```python
from build123d import *

# Parameters (mm, degrees)
SKETCH1_W           = 105
SKETCH1_H           = 530
BOSS_EXTRUDE1_DEPTH = 7.5
LPATTERN1_COUNT     = 4
LPATTERN1_PITCH     = 25


# Read off the part's stored shape, not the designer's step: Mirror1
with BuildPart() as part:
    # Sketch1 → Boss-Extrude1 (new, symmetric)
    with BuildSketch(Plane(origin=(0, 0, 0), x_dir=(0, -1, 0), z_dir=(0, 0, 1))):
        Rectangle(SKETCH1_W, SKETCH1_H)
    extrude(amount=BOSS_EXTRUDE1_DEPTH, both=True)

    # Sketch2 → Cut-Loft1 section 0
    with BuildSketch(Plane.XY.offset(-4.5)):
        with BuildLine():
            Line((265, 47.5), (265, 32.5))
            Line((265, 32.5), (260, 32.5))
            ThreePointArc((260, 32.5), (252.5, 40), (260, 47.5))
            Line((260, 47.5), (265, 47.5))
        make_face()
    # Sketch3 → Cut-Loft1 section 1
    with BuildSketch(Plane.XY.offset(7.5)):
        with BuildLine():
            Line((265, 46), (265, 34))
            Line((265, 34), (260, 34))
            ThreePointArc((260, 34), (254, 40), (260, 46))
            Line((260, 46), (265, 46))
        make_face()
    cut_loft1 = loft(mode=Mode.SUBTRACT)

    # LPattern1: Cut-Loft1 ×4
    with Locations(*[(0, -i * LPATTERN1_PITCH, 0) for i in range(1, LPATTERN1_COUNT)]):
        add(cut_loft1, mode=Mode.SUBTRACT)

    # Mirror1
    split(bisect_by=Plane(origin=(0, 0, 0), x_dir=(0, 0, 1), z_dir=(1, 0, 0)), keep=Keep.TOP)

    # Mirror1 2: part across plane


with BuildPart() as part_1:
    add(part.part)
    add(part.part.mirror(Plane(origin=(0, 0, 0), x_dir=(0, 0, 1), z_dir=(1, 0, 0))))


solid = part_1.part
```
The model under review builds one solid part; all positions refer to its coordinate system, in mm. Give positions to 0.01 mm unless a question says otherwise; leave off trailing zeros. Write each loop counter-clockwise with the first axis right and the second up, starting at its lowest first coordinate (ties: lowest second). Pieces come first, ordered by that corner, then holes. Notation, with made-up numbers: (35.5, -24.5) -> (60.5, -24.5) arc R27 ccw to (60.5, -8.5) -> close; hole circle Ø2 at (-14, 37). An arc over 180 degrees is marked (long way). Answer in a Markdown table with one row per item.
1) For L1, parallel to X at y = -41.5, z = -4.25; L2, parallel to X at y = -39.5, z = 0.75, list the stretches that pass through material, from the lowest coordinate up. Write a range as [from, to].
Worked answers:
| item | result |
|---|---|
| L1 | [-256.32, 256.32] |
| L2 | [-254.84, 254.84] |
2) Mouldability with a two-part tool opening along Y and no side actions: class faces 1 (the flat face through (4, -52.5, 0)), 2 (the flat face through (-260, 15, -4.5)), 3 (the flat face through (-4, 1, -7.5)), 4 (the conical face through (-253.26, 14.85, 1.58)) as +Y half, -Y half, draft (parallel to the pull), parting line (faces both ways), or undercut.
Worked answers:
| item | result |
|---|---|
| face 1 | -Y half |
| face 2 | undercut |
| face 3 | draft |
| face 4 | undercut |
3) Clearance check with flat-ended pins moving along their axes: P1, Ø6, axis at x = -257.5, y = -33.5, coming from the +Z side; P2, Ø10, axis at x = -260.5, y = -7.5, coming from the +Z side. State where each tip first meets the part, or that it passes through.
Worked answers:
| item | result |
|---|---|
| P1 | z = -4.5 |
| P2 | z = 7.5 |
4) Add section A-A on y = -35. State the section outline as (x, z) points, plus the area to 3 significant figures.
Worked answers:
| item | result |
|---|---|
| outline | (-265, -7.5) -> (265, -7.5) -> (265, -4.5) -> (252.5, -4.5) -> (254, 7.5) -> (-254, 7.5) -> (-252.5, -4.5) -> (-265, -4.5) -> close |
| area | 7,670 mm² |
